from build123d import *

# Parameters (mm, degrees)
F0_W      = 15
F0_H      = 5
F2_R      = 20
F3_R      = 10
F4_R      = 3
F5_DEPTH  = 100
F7_START  = -25
F6_R      = 6
F7_DEPTH  = 75
F8_R      = 1
F9_R      = 2
F11_DEPTH = 25


with BuildPart() as f1:
    # F0 (on Front) → F1 (revolve)
    with BuildSketch(Plane.XZ):
        with BuildLine():
            Line((0, 0), (0, -60))
            ThreePointArc((0, -60), (20.8180621376, -57.0528159674), (40, -48.4428877022))
            Line((40, -48.4428877022), (40, -30))
            Line((40, -30), (15, -30))
            Line((15, -30), (15, 0))
            Line((15, 0), (0, 0))
        make_face()
        with Locations((7.5, 2.5)):
            Rectangle(F0_W, F0_H)
    revolve(axis=Axis((0, 0, -30), (0, 0, 1)))

    # F2
    f2_edges = [f1.edges().sort_by_distance(p)[0] for p in [
        (-15, 0, -30),
    ]]
    fillet(f2_edges, radius=F2_R)

    # F3
    f3_edges = [f1.edges().sort_by_distance(p)[0] for p in [
        (-40, 0, -48.442888),
        (-40, 0, -30),
    ]]
    fillet(f3_edges, radius=F3_R)

    # F4 (on Top) → F5 (cut, symmetric)
    with BuildSketch(Plane.XY):
        Circle(F4_R)
    extrude(amount=F5_DEPTH, both=True, mode=Mode.SUBTRACT)

    # F6 (on Top) → F7 (cut)
    with BuildSketch(Plane.XY.offset(F7_START)):
        Circle(F6_R)
    extrude(amount=-F7_DEPTH, mode=Mode.SUBTRACT)

    # F8
    f8_edges = [f1.edges().sort_by_distance(p)[0] for p in [
        (-6, 0, -25),
    ]]
    fillet(f8_edges, radius=F8_R)

    # F9
    f9_edges = [f1.edges().sort_by_distance(p)[0] for p in [
        (-6, 0, -59.759615),
    ]]
    fillet(f9_edges, radius=F9_R)

    # F10 (on Front) → F11 (cut, symmetric)
    with BuildSketch(Plane.XZ):
        Polygon((-50, -8.8163490354), (50, 8.8163490354), (-50, 8.8163490354), align=None)
    extrude(amount=F11_DEPTH, both=True, mode=Mode.SUBTRACT)


solid = f1.part
The listing builds one solid part. Answer for the finished solid, in the listing's coordinates (mm). A direction names the side the tool comes from. Give positions to 0.01 mm unless a question says otherwise; leave off trailing zeros. Use a Markdown table: item, result.
(1) Find the intervals of material crossed by probe 1 along Y at (x, z) = (0, -45.5); probe 2 along Y at (x, z) = (0, -45); probe 3 along X at (y, z) = (0, -15), in increasing order. Write a range as from..to.
Return value:
| item | result |
|---|---|
| probe 1 | -39.59..-6, 6..39.59 |
| probe 2 | -39.72..-6, 6..39.72 |
| probe 3 | -15.64..-3, 3..15.64 |
(2) Determine the mould class of faces 1 (the cylindrical face through (14.307, 4.506, -4.994)), 2 (the flat face through (0, -4, 0)), 3 (the cylindrical face through (-3, 0, -12)) for opening direction X: released by +X, released by -X, zero draft, split by the parting line, or undercut.
Return value:
| item | result |
|---|---|
| face 1 | split by the parting line |
| face 2 | released by -X |
| face 3 | undercut |
(3) Flat-ended cylindrical pins translate along their axes: P1, Ø5, axis at x = 10, z = -31.5, coming from the +Y side; P2, Ø7, axis at x = 0, y = 0, coming from the +Z side; P3, Ø6, axis at x = -8.5, y = -26.5, coming from the +Z side. Find the tip coordinate at first contact, or state that the pin passes through.
Return value:
| item | result |
|---|---|
| P1 | y = 37.08 |
| P2 | z = 0.62 |
| P3 | z = -27.22 |
(4) For faces 4 (the cylindrical face through (38.153, 12.015, -41.1)), 5 (the cylindrical face through (-0.78, 5.95, -41.56)), determine the directions among +Z, -Z, +X, -X, +Y, -Y from which every point of the face is accessible in a straight line to the end or side of a thin tool.
Return value:
| item | result |
|---|---|
| face 4 | +Z, -Z |
| face 5 | -Z |
